Read the model definition and answer for the solid it produces. Units are mm, in the model's axes. Give positions to 0.01 mm unless a question says otherwise; leave off trailing zeros. Order: outer loops, then holes, each group sorted by start corner. A loop starts at its lowest first (then second) coordinate and runs counter-clockwise, first axis right, second up. Notation, with made-up numbers: (37.5, 17) - (79.5, 17) arc R23 cw to (79.5, 30) - close; hole circle Ø2 at (26.5, 4.25). An arc over 180 degrees is marked (long way). Write item = value, one per line.
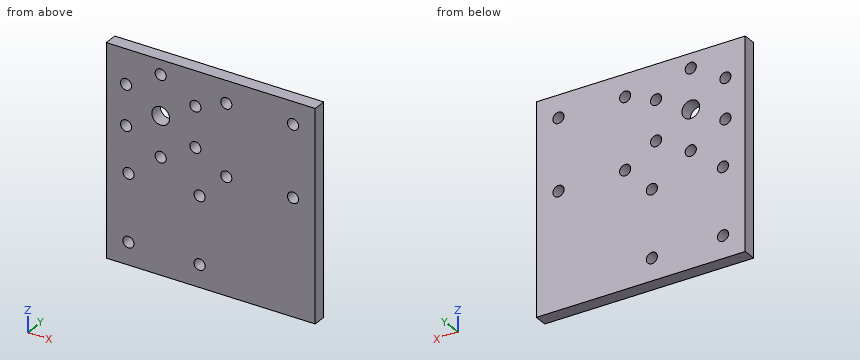
```python
from build123d import *

# Parameters (mm, degrees)
SKETCH1_W                   = 47
SKETCH1_H                   = 47
BOSS_EXTRUDE1_DEPTH         = 3
TAP_DRILL_FOR_M3X0_5_TAP1_D = 2.5
TAP_DRILL_FOR_M3X0_5_TAP2_D = 2.5
F_4_0_4_DIAMETER_HOLE1_D    = 4


with BuildPart() as part:
    # Sketch1 → Boss-Extrude1 (new body)
    with BuildSketch(Plane(origin=(0, 0, 0), x_dir=(1, 0, 0), z_dir=(0, 1, 0))):
        with Locations((10.5, -11)):
            Rectangle(SKETCH1_W, SKETCH1_H)
    extrude(amount=BOSS_EXTRUDE1_DEPTH)

    # Tap Drill for M3x0.5 Tap1 (through all)
    with Locations(Plane(origin=(0, 3, 0), x_dir=(1, 0, 0), z_dir=(0, 1, 0))):
        with Locations((-8, 7.5), (8, 7.5), (8, -7.5), (-8, -7.5), (14, -13.5), (29, -13.5), (29, -29.5), (14, -29.5)):
            Hole(TAP_DRILL_FOR_M3X0_5_TAP1_D / 2)

    # Tap Drill for M3x0.5 Tap2 (through all)
    with Locations(Plane(origin=(0, 3, 0), x_dir=(1, 0, 0), z_dir=(0, 1, 0))):
        with Locations((-0.75, -13.25), (-8.544228634, -17.75), (-8.544228634, -26.75), (-0.75, -31.25), (7.044228634, -26.75), (7.044228634, -17.75)):
            Hole(TAP_DRILL_FOR_M3X0_5_TAP2_D / 2)

    # Ø4.0 (4) Diameter Hole1 (through all)
    with Locations(Plane(origin=(0, 3, 0), x_dir=(1, 0, 0), z_dir=(0, 1, 0))):
        with Locations((-0.75, -22.25)):
            Hole(F_4_0_4_DIAMETER_HOLE1_D / 2)


solid = part.part
```
1. Section C-C (y = 1) is taken. Count the separate pieces of the cut face and the enclosed holes in it, and give its area (3 significant figures).
Recorded:
separate_pieces = 1
enclosed_holes = 15
area = 2,130 mm^2
2. Straight lines are drawn through the part: L1, parallel to Z at x = -0.75, y = 0.85; L2, parallel to X at y = 1.9, z = -7.5; L3, parallel to X at y = 2, z = 29.5. For each, find the intervals that lie inside material, in ascending order. Write a range as [from, to].
Recorded:
L1 = [-12.5, 12], [14.5, 20.25], [24.25, 30], [32.5, 34.5]
L2 = [-13, -9.25], [-6.75, 6.75], [9.25, 34]
L3 = [-13, 12.75], [15.25, 27.75], [30.25, 34]
3. Section D-D (x = -8) is taken. Determine the outline of the cut face in (y, z), and give its area (3 significant figures).
Recorded:
outline = (0, -12.5) - (3, -12.5) - (3, -8.75) - (0, -8.75) - close; (0, -6.25) - (3, -6.25) - (3, 6.25) - (0, 6.25) - close; (0, 8.75) - (3, 8.75) - (3, 16.62) - (0, 16.62) - close; (0, 18.88) - (3, 18.88) - (3, 25.62) - (0, 25.62) - close; (0, 27.88) - (3, 27.88) - (3, 34.5) - (0, 34.5) - close
area = 112 mm^2
4. Section B-B (z = 17.75) is taken. Determine the outline of the cut face in (x, y).
Recorded:
outline = (-13, 0) - (-9.79, 0) - (-9.79, 3) - (-13, 3) - close; (-7.29, 0) - (5.79, 0) - (5.79, 3) - (-7.29, 3) - close; (8.29, 0) - (34, 0) - (34, 3) - (8.29, 3) - close
5. Section A-A (x = 14) is taken. Determine the outline of the cut face in (y, z), and give its area (3 significant figures).
Recorded:
outline = (0, -12.5) - (3, -12.5) - (3, 12.25) - (0, 12.25) - close; (0, 14.75) - (3, 14.75) - (3, 28.25) - (0, 28.25) - close; (0, 30.75) - (3, 30.75) - (3, 34.5) - (0, 34.5) - close
area = 126 mm^2
